```python
from build123d import *

# Parameters (mm, degrees)
ESQUISSE1_R        = 19
ESQUISSE1_R_2      = 1.5
BOSS_EXTRU_2_DEPTH = 6


with BuildPart() as part:
    # Esquisse1 → Boss.-Extru.2 (new body)
    with BuildSketch(Plane.XY):
        Circle(ESQUISSE1_R)
        with Locations((-0.493805045, 13.991288596)):
            Circle(ESQUISSE1_R_2, mode=Mode.SUBTRACT)
        with Locations((12.363713879, -6.567996584)):
            Circle(ESQUISSE1_R_2, mode=Mode.SUBTRACT)
        with Locations((-11.869908833, -7.423292012)):
            Circle(ESQUISSE1_R_2, mode=Mode.SUBTRACT)
        with BuildLine():
            ThreePointArc((-2.815595301, 11.717131607), (-0.379171731, 10.743310886), (1.982535482, 11.886475637))
            ThreePointArc((1.982535482, 11.886475637), (3.751818189, 12.953817976), (5.806908291, 12.738909534))
            ThreePointArc((5.806908291, 12.738909534), (11.869908833, 7.423292012), (13.995505264, -0.354728625))
            ThreePointArc((13.995505264, -0.354728625), (13.289218046, -2.296567787), (11.555131282, -3.420188746))
            ThreePointArc((11.555131282, -3.420188746), (9.493566014, -5.043283091), (9.302722122, -7.66016391))
            ThreePointArc((9.302722122, -7.66016391), (9.342426349, -9.72607885), (8.128765127, -11.398384864))
            ThreePointArc((8.128765127, -11.398384864), (0.493805045, -13.991288596), (-7.304956633, -11.943098785))
            ThreePointArc((-7.304956633, -11.943098785), (-8.633495068, -10.360516531), (-8.739535981, -8.296942861))
            ThreePointArc((-8.739535981, -8.296942861), (-9.114394283, -5.700027795), (-11.285257604, -4.226311727))
            ThreePointArc((-11.285257604, -4.226311727), (-13.094244538, -3.227739126), (-13.935673418, -1.34052467))
            ThreePointArc((-13.935673418, -1.34052467), (-12.363713879, 6.567996584), (-6.690548632, 12.29782741))
            ThreePointArc((-6.690548632, 12.29782741), (-4.655722978, 12.657084318), (-2.815595301, 11.717131607))
        make_face(mode=Mode.SUBTRACT)
    extrude(amount=BOSS_EXTRU_2_DEPTH)


solid = part.part
```
The model under review builds one solid part; all positions refer to its coordinate system, in mm. A direction names the side the tool comes from. Give positions to 0.01 mm unless a question says otherwise; leave off trailing zeros. Write each loop counter-clockwise with the first axis right and the second up, starting at its lowest first coordinate (ties: lowest second). Pieces come first, ordered by that corner, then holes. Notation, with made-up numbers: M 0,10 L 23,10 A10 cw 23,18 Z; hole C 83,85 d8. An arc over 180 degrees is marked long. Answer in a Markdown table with one row per item.
Item 1: Add section D-D on y = 17. Give the boundary of the cut face in (x, z), plus the area to 3 significant figures.
Check sheet entries:
| item | result |
|---|---|
| outline | M -8.49,0 L 8.49,0 L 8.49,6 L -8.49,6 Z |
| area | 102 mm2 |
Item 2: Add section C-C on x = 5. Give the boundary of the cut face in (y, z).
Check sheet entries:
| item | result |
|---|---|
| outline | M -18.33,0 L -13.08,0 L -13.08,6 L -18.33,6 Z; M 12.99,0 L 18.33,0 L 18.33,6 L 12.99,6 Z |
Item 3: For line 1 along X through (y, z) = (-7, 1.45); line 2 along X through (y, z) = (-9, 5.1); line 3 along Y through (x, z) = (-12.5, 4.7), list the stretches that pass through material, from the lowest coordinate up.
Check sheet entries:
| item | result |
|---|---|
| line 1 | -17.66 to -13.31, -10.43 to -8.65, 9.14 to 10.93, 13.8 to 17.66 |
| line 2 | -16.73 to -8.85, 9.48 to 16.73 |
| line 3 | -14.31 to -8.78, -6.06 to -3.74, 6.3 to 14.31 |
Item 4: For P1, Ø5, axis at x = 12.36, y = -6.57, coming from the -Z side; P2, Ø1.5, axis at y = 14, z = 4, coming from the +X side; P3, Ø1.5, axis at x = -1.5, z = 1, coming from the -Y side, all flat-tipped, find the tip position at first contact; note any pin that passes through.
Check sheet entries:
| item | result |
|---|---|
| P1 | z = 0 |
| P2 | x = 13.62 |
| P3 | y = -18.99 |
Item 5: Tool access review of faces 4 (the face through (11.81, 7.52, 2.96)), 5 (the face through (12, -4, 0)): name each direction out of +Z, -Z, +X, -X, +Y, -Y from which nothing blocks a thin tool from reaching the whole face with its end or side.
Check sheet entries:
| item | result |
|---|---|
| face 4 | +Z, -Z |
| face 5 | -Z, +X, -X, +Y, -Y |
Item 6: Add section A-A on x = 0. Give the boundary of the cut face in (y, z), plus the area to 3 significant figures.
Check sheet entries:
| item | result |
|---|---|
| outline | M -19,0 L -14,0 L -14,6 L -19,6 Z; M 10.78,0 L 12.57,0 L 12.57,6 L 10.78,6 Z; M 15.41,0 L 19,0 L 19,6 L 15.41,6 Z |
| area | 62.3 mm2 |
Item 7: Add section B-B on z = 4.25. Give the boundary of the cut face in (x, y).
Check sheet entries:
| item | result |
|---|---|
| outline | C 0,0 d38; hole M -13.94,-1.34 A3.25 ccw -11.29,-4.23 A3.25 cw -8.74,-8.3 A3.25 ccw -7.3,-11.94 A14 ccw 8.13,-11.4 A3.25 ccw 9.3,-7.66 A3.25 cw 11.56,-3.42 A3.25 ccw 14,-0.35 A14 ccw 5.81,12.74 A3.25 ccw 1.98,11.89 A3.25 cw -2.82,11.72 A3.25 ccw -6.69,12.3 A14 ccw Z; hole C -11.87,-7.42 d3; hole C -0.49,13.99 d3; hole C 12.36,-6.57 d3 |
Item 8: Draft analysis for pull direction Y (two halves, no side actions). For faces 1 (the face through (8.767, -16.856, 2.958)), 2 (the face through (0.608, -13.987, 2.958)), 3 (the face through (12, -4, 6)), state which applies: +Y half, -Y half, draft (parallel to the pull), parting line (faces both ways), or undercut.
Check sheet entries:
| item | result |
|---|---|
| face 1 | parting line |
| face 2 | undercut |
| face 3 | draft |
